Autodesk Inventor part; units mm, degrees
ref_plane "YZ Plane" through (0, 0, 0) normal (1, 0, 0) x (0, 1, 0)
ref_plane "XZ Plane" through (0, 0, 0) normal (0, 1, 0) x (-1, 0, 0)
ref_plane "XY Plane" through (0, 0, 0) normal (0, 0, 1) x (1, 0, 0)
sketch "Sketch1" plane through (0, 0, 0) normal (0, 1, 0) x (-1, 0, 0)
  line L0 (0, 0) -> (0, 13.5)
  line L1 (0, 13.5) -> (1.75, 13.5)
  line L2 (1.75, 13.5) -> (1.75, 4)
  line L3 (0, 0) -> (3.25, 0.75)
  line L4 (1.75, 4) -> (3.25, 0.75)
  dimension "d0" = 13.5
  dimension "d1" = 1.75
  dimension "d2" = 3.25
  dimension "d4" = 0.75
  dimension "d5" = 9.5
revolve "Revolution1" add sketch "Sketch1" angle 360 about axis through (0, 0, 0) along (0, 0, 1)
ref_plane "Work Plane1" through (0, 0, 0) normal (0, 0, 1) x (1, 0, 0)
sketch "Sketch2" plane through (0, 0, 0) normal (0, 0, 1) x (1, 0, 0)
  line L0 (0.5, 3.2113) -> (0.5, -3.2113)
  line L1 (-0.5, 3.2113) -> (-0.5, -3.2113)
  circle A0 centre (0, 0) radius 3.25
  dimension "d8" = 1
  dimension "d9" = 0.5
extrude "Extrusion1" cut sketch "Sketch2" along normal blind 1.25 contours L0 A0 L1
thread "Thread1"
fillet "Fillet1" radius 0.5 1 edges at (1.75, 0, 13.5)
properties part number "Screw"
The listing builds one solid part. Answer for the finished solid, in the listing's coordinates (mm). A direction names the side the tool comes from. Give positions to 0.01 mm unless a question says otherwise; leave off trailing zeros. Loops run counter-clockwise (first coordinate to the right, second up) from the corner with the lowest first, then second, coordinate; pieces in that order, holes last. Notation, with made-up numbers: M -39.75,-39 L 17.25,-39 A19 cw 17.25,-10 Z; hole C -30,61.25 d4. An arc over 180 degrees is marked long. One line per item, written item: value.
1. Section B-B on y = 0 is taken. Determine the outline of the cut face in (x, z), plus the area to 3 significant figures.
Found:
outline: M -3.25,0.75 L -0.5,0.12 L -0.5,1.25 L 0.5,1.25 L 0.5,0.12 L 3.25,0.75 L 1.75,4 L 1.75,13 A0.5 ccw 1.25,13.5 L -1.25,13.5 A0.5 ccw -1.75,13 L -1.75,4 Z
area: 50.6 mm^2
2. Section D-D on z = 2 is taken. Determine the outline of the cut face in (x, y), plus the area to 3 significant figures.
Found:
outline: C 0,0 d5.35
area: 22.4 mm^2
3. Section C-C on z = 6 is taken. Determine the outline of the cut face in (x, y).
Found:
outline: C 0,0 d3.5
4. Find the intervals of material crossed by probe 1 along Y at (x, z) = (0, 6); probe 2 along Z at (x, y) = (1.5, 1.25); probe 3 along Y at (x, z) = (0.5, 1.5), in increasing order.
Found:
probe 1: -1.75 to 1.75
probe 2: 0.45 to 3.56
probe 3: -2.86 to 2.86
5. For faces 4 (the face through (1.586, -0.031, 0.366)), 5 (the face through (-1.617, -0.67, 8.437)), 6 (the face through (-0.5, 0, 1)), determine the directions among +Z, -Z, +X, -X, +Y, -Y from which every point of the face is accessible in a straight line to the end or side of a thin tool.
Found:
face 4: -Z, +X
face 5: +Z
face 6: -Z, +Y, -Y
6. Section A-A on x = 0 is taken. Determine the outline of the cut face in (y, z).
Found:
outline: M -3.02,1.25 L 3.02,1.25 L 1.75,4 L 1.75,13 A0.5 ccw 1.25,13.5 L -1.25,13.5 A0.5 ccw -1.75,13 L -1.75,4 Z
7. For a pull along X with two mould halves and no side action, classify faces 1 (the face through (-1.588, 0.031, 0.367)), 2 (the face through (0.5, 0, 1)), 3 (the face through (0, 0, 13.5)) as pulls with the +X half, pulls with the -X half, needs draft (parallel to the pull), parting line crosses it, or undercut.
Found:
face 1: pulls with the -X half
face 2: undercut
face 3: needs draft
8. Each of these flat-tipped pins is pushed along its axis until it touches: P1, Ø2, axis at y = 1.5, z = 11.5, coming from the -X side; P2, Ø0.9, axis at y = -1.5, z = 0.5, coming from the -X side; P3, Ø0.5, axis at x = 0, y = -1, coming from the -Z side. Where does it stop, or does it pass through?
Found:
P1: x = -1.68
P2: x = -3.05
P3: z = 1.25
